```python
from build123d import *

# Parameters (mm, degrees)
F0_W     = 33.957731
F0_H     = 25.119421
F1_DEPTH = 25.4
F3_D     = 12.7
F3_DEPTH = 25.4


with BuildPart() as f1:
    # F0 (on Front) → F1 (new body)
    with BuildSketch(Plane.XZ):
        with Locations((-29.305988, 27.445291)):
            Rectangle(F0_W, F0_H)
    extrude(amount=F1_DEPTH)

    # F3
    with Locations(Plane.XZ.offset(25.4)):
        with Locations((-31.166686, 28.375639)):
            Hole(F3_D / 2, depth=F3_DEPTH)


solid = f1.part
```
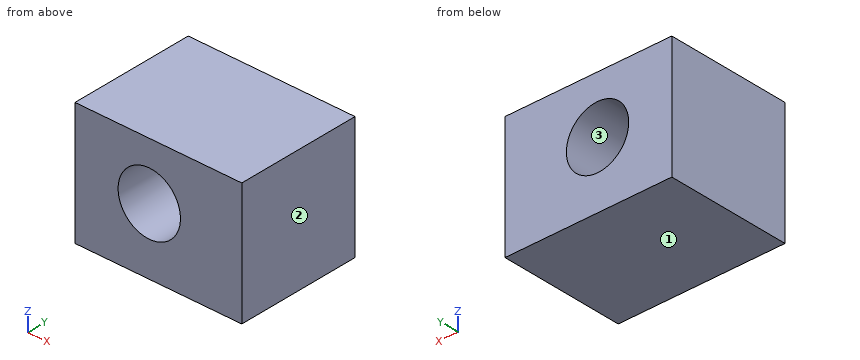
For this review, take the finished solid that the model builds, in its own axes (mm). Face numbers are marked on the shaded views. Coordinates: 2 decimals unless noted, no trailing zeros. Order: outer loops, then holes, each group sorted by start corner. A loop starts at its lowest first (then second) coordinate and runs counter-clockwise, first axis right, second up. Notation, with made-up numbers: (15.25, -29.5) - (57.25, -29.5) arc R21 ccw to (57.25, -8.5) - close; hole circle Ø3 at (-18.5, 64.5). An arc over 180 degrees is marked (long way). Answer as a JSON object with one key per item and string values. Group by question number.
1. The part is to be moulded in two halves that separate along X. For the marked faces 1, 2 and 3, say which applies: pulls with the +X half, pulls with the -X half, needs draft (parallel to the pull), parting line crosses it, or undercut.
2. We need section C-C on y = -12.25. State the section outline as (x, z) points (3 decimals).
3. We need section A-A on z = 29.5. State the section outline as (x, y) points.
4. We need section B-B on x = -35. State the section outline as (y, z) points (3 decimals), then the cut area to 3 significant figures.
5. For probe 1 along Z at (x, y) = (-32, -4.5) (3 decimals); probe 2 along Z at (x, y) = (-29, -11.25) (3 decimals); probe 3 along X at (y, z) = (-9.75, 27.25), list the stretches that pass through material, from the lowest coordinate up.
6. Clearance check with a flat-ended pin moving along its axis: P1, Ø10, axis at x = -31.17, z = 28.38, coming from the -Y side. State where the tip first meets the part, or that it passes through.
Final values:
{
 "1": {"face 1": "needs draft", "face 2": "pulls with the +X half", "face 3": "undercut"},
 "2": {"outline": "(-46.285, 14.886) - (-12.327, 14.886) - (-12.327, 40.005) - (-46.285, 40.005) - close; hole circle Ø12.7 at (-31.167, 28.376)"},
 "3": {"outline": "(-46.28, -25.4) - (-37.42, -25.4) - (-37.42, 0) - (-46.28, 0) - close; (-24.92, -25.4) - (-12.33, -25.4) - (-12.33, 0) - (-24.92, 0) - close"},
 "4": {"outline": "(-25.4, 14.886) - (0, 14.886) - (0, 23.313) - (-25.4, 23.313) - close; (-25.4, 33.438) - (0, 33.438) - (0, 40.005) - (-25.4, 40.005) - close", "area": "381 mm²"},
 "5": {"probe 1": "14.886 to 22.081, 34.671 to 40.005", "probe 2": "14.886 to 22.407, 34.345 to 40.005", "probe 3": "-46.28 to -37.42, -24.92 to -12.33"},
 "6": {"P1": "through"}
}
